Geometry check sheet. Reference: drawing and pictorial views, mm from the part's lowest x, y, z. A direction names the side the tool comes from. Give positions to 0.01 mm unless a question says otherwise; leave off trailing zeros. Order: outer loops, then holes, each group sorted by start corner. A loop starts at its lowest first (then second) coordinate and runs counter-clockwise, first axis right, second up. Notation, with made-up numbers: M -11.75,35 L 30.25,35 A15 cw 30.25,39 Z; hole C 72,21 d10. An arc over 180 degrees is marked long. Use CSV: the item, a comma, the result in double quotes. Start each with the question number.
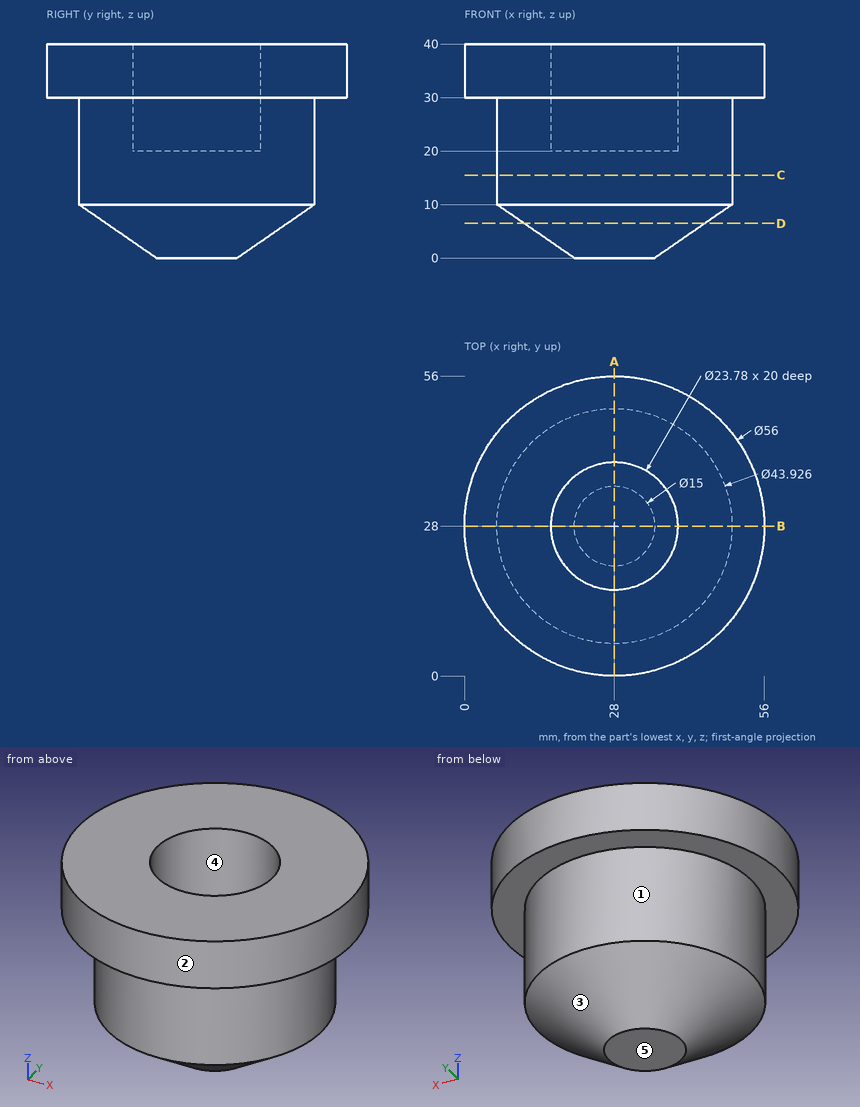
(1) Sectioned sample at A-A on x = 28. Record the cut outline in (y, z), then the cut area to 3 significant figures.
(2) Go/stop test with flat-tipped pins: P1, Ø1.5, axis at x = 23.5, y = 32, coming from the -Z side; P2, Ø5, axis at y = 10.5, z = 21.5, coming from the +X side; P3, Ø2, axis at x = 50.5, z = 33, coming from the +Y side; P4, Ø7, axis at x = 29, y = 27, coming from the +Z side. Record where each tip stops, or that it passes through.
(3) Draft check along Y on the marked faces 3, 4 and 5. Enter one of: +Y half, -Y half, draft (parallel to the pull), parting line (faces both ways), or undercut.
(4) Thickness scan on line 1 (Y direction, x = 28, z = 26.5); line 2 (Y direction, x = 28, z = 35); line 3 (Z direction, x = 5, y = 12.5). Record the ranges inside material, lowest first.
(5) Sectioned sample at D-D on z = 6.5. Record the cut outline in (x, y), then the cut area to 3 significant figures.
(6) Access from +Z, -Z, +X, -X, +Y, -Y to the whole of each face (thin tool, end or side, straight path). Record for the marked faces 1 and 2.
(7) Sectioned sample at C-C on z = 15.5. Record the cut outline in (x, y).
Responses:
1,outline,"M 0,30 L 6.04,30 L 6.04,10 L 20.5,0 L 35.5,0 L 49.96,10 L 49.96,30 L 56,30 L 56,40 L 39.89,40 L 39.89,20 L 16.11,20 L 16.11,40 L 0,40 Z"
1,area,"1,260 mm2"
2,P1,"z = 0"
2,P2,"x = 44.04"
2,P3,"y = 45.94"
2,P4,"z = 20"
3,face 3,"parting line"
3,face 4,"undercut"
3,face 5,"draft"
4,line 1,"6.04 to 16.11, 39.89 to 49.96"
4,line 2,"0 to 16.11, 39.89 to 56"
4,line 3,"30 to 40"
5,outline,"C 28,28 d33.8"
5,area,"897 mm2"
6,face 1,"-Z"
6,face 2,"+Z, -Z"
7,outline,"C 28,28 d43.93"
